from build123d import *

# Parameters (mm, degrees)
F0_R     = 160
F0_R_2   = 42.35
F0_R_3   = 25
F1_DEPTH = 110
F2_DEPTH = 35
F3_SIZE  = 80


with BuildPart() as f1:
    # F0 (on Front) → F1 (new body)
    with BuildSketch(Plane.XZ):
        Circle(F0_R)
        Circle(F0_R_2, mode=Mode.SUBTRACT)
        Circle(F0_R_2)
        Circle(F0_R_3, mode=Mode.SUBTRACT)
    extrude(amount=F1_DEPTH)

    # F0 (on Front) → F2 (join)
    with BuildSketch(Plane.XZ):
        Circle(F0_R_2)
        Circle(F0_R_3, mode=Mode.SUBTRACT)
    extrude(amount=-F2_DEPTH)

    # F3
    f3_edges = [f1.edges().sort_by_distance(p)[0] for p in [
        (-160, -110, 0),
    ]]
    chamfer(f3_edges, length=F3_SIZE)


solid = f1.part
Work out the finished part from the listing and answer in its coordinate system (mm). A direction names the side the tool comes from. Round coordinates to 2 decimals unless told otherwise and drop trailing zeros. Write each loop counter-clockwise with the first axis right and the second up, starting at its lowest first coordinate (ties: lowest second). Pieces come first, ordered by that corner, then holes. Notation, with made-up numbers: (-18.75, 69) -> (18.25, 69) arc R10 ccw to (18.25, 82) -> close; hole circle Ø6 at (4, 26). An arc over 180 degrees is marked (long way). Answer as CSV lines item,"result". Start each with the question number.
(1) Each of these flat-tipped pins is pushed along its axis until it touches: pin 1 (12 mm diameter, centred on x = -11, z = -104, fed in from +Y); pin 2 (12 mm diameter, centred on y = -88.5, z = -115.5, fed in from +X); pin 3 (3 mm diameter, centred on y = -59.5, z = -30.5, fed in from +X); pin 4 (4 mm diameter, centred on y = -5, z = 98, fed in from -X). Where does it stop, or does it pass through?
(2) Find the intervals of material crossed by probe 1 along Z at (x, y) = (0, -12.5); probe 2 along Z at (x, y) = (0, -41); probe 3 along Y at (x, z) = (-40, -100.5), in increasing order.
(3) The part is cut by section B-B, the plane x = 0. Give the vertices of the cut face in (y, z), then the cut area to 3 significant figures.
(4) The mould has two halves that part along X. Classify faces 1 (the conical face through (-18.2, -106.1, -81.9)), 2 (the cylindrical face through (23.846, -36.485, 7.509)), 3 (the flat face through (17, -110, 19)): +X half, -X half, draft (parallel to the pull), parting line (faces both ways), or undercut.
(5) A tool of negligible diameter and unlimited length cuts with its end or side. For faces 4 (the flat face through (33, 0, -33)), 5 (the cylindrical face through (-34.685, -14.79, -156.195)), from which of +Z, -Z, +X, -X, +Y, -Y can it reach the whole face along a straight path? Write none if from no direction.
(6) The part is cut by section A-A, the plane z = 0. Give the vertices of the cut face in (x, y), then the cut area to 3 significant figures.
(7) The part is cut by section C-C, the plane y = -78.5. Give the vertices of the cut face in (x, z), then the cut area to 3 significant figures.
Output values:
1,pin 1,"stops at y = 0"
1,pin 2,"passes through"
1,pin 3,"stops at x = 128.47"
1,pin 4,"stops at x = -128"
2,probe 1,"z = -160 to -25, 25 to 160"
2,probe 2,"z = -149 to -25, 25 to 149"
2,probe 3,"y = -81.83 to 0"
3,outline,"(-110, -80) -> (-30, -160) -> (0, -160) -> (0, -42.35) -> (35, -42.35) -> (35, -25) -> (-110, -25) -> close; (-110, 25) -> (35, 25) -> (35, 42.35) -> (0, 42.35) -> (0, 160) -> (-30, 160) -> (-110, 80) -> close"
3,area,"24,500 mm²"
4,face 1,"parting line"
4,face 2,"undercut"
4,face 3,"draft"
5,face 4,"+Y"
5,face 5,"+Y, -Y"
6,outline,"(-160, -30) -> (-80, -110) -> (-25, -110) -> (-25, 35) -> (-42.35, 35) -> (-42.35, 0) -> (-160, 0) -> close; (25, -110) -> (80, -110) -> (160, -30) -> (160, 0) -> (42.35, 0) -> (42.35, 35) -> (25, 35) -> close"
6,area,"24,500 mm²"
7,outline,"circle Ø223 at (0, 0); hole circle Ø50 at (0, 0)"
7,area,"37,100 mm²"
